Job drawing, mm, ordinate dimensions from the low corner. One solid piece. Coordinates: 2 decimals unless noted, no trailing zeros. Loops run counter-clockwise (first coordinate to the right, second up) from the corner with the lowest first, then second, coordinate; pieces in that order, holes last. Notation, with made-up numbers: (-29.5, 75.5) -> (11.5, 75.5) arc R6 ccw to (11.5, 86.5) -> close; hole circle Ø1 at (57, -36). An arc over 180 degrees is marked (long way). Use one line per item in the form item = value. Start each with the question number.
(1) Drill centre lines: L1, parallel to X at y = 21, z = 2.4; L2, parallel to Z at x = 17, y = 88. Where is each one in solid material? Low to high. Write a range as [from, to].
(2) Pin check, flat tips, straight feed: P1, Ø12, axis at x = 16, y = 41.5, coming from the +Z side; P2, Ø1, axis at x = 39.5, z = 3, coming from the +Y side; P3, Ø0.6, axis at x = 39.5, z = 2.5, coming from the -Y side. Stop position of each tip, or through.
(3) Band-saw the part on A-A on z = 2.85. Give the cut face in (x, y), then the cut area to 3 significant figures.
(4) Band-saw the part on B-B on y = 89.5. Give the cut face in (x, z).
(5) Band-saw the part on C-C on x = 25. Give the cut face in (y, z), then the cut area to 3 significant figures.
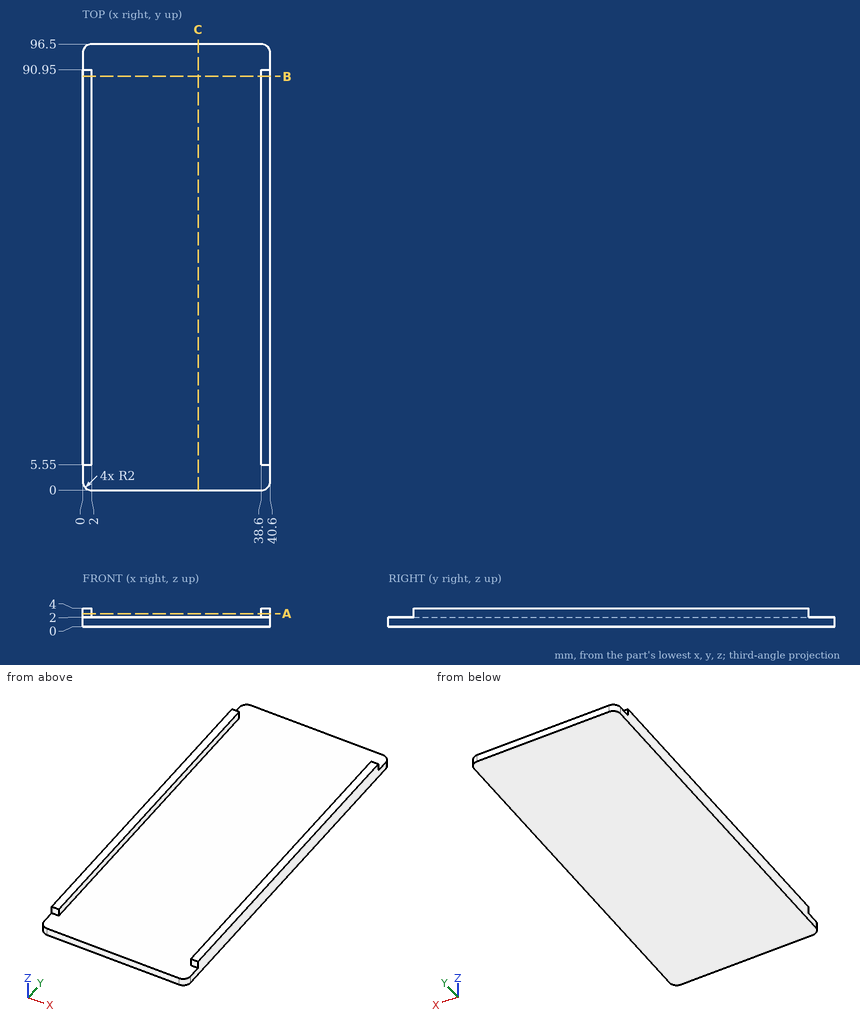
A:
q1.L1 = [0, 2], [38.6, 40.6]
q1.L2 = [0, 2]
q2.P1 = 2
q2.P2 = 90.95
q2.P3 = 5.55
q3.outline = (0, 5.55) -> (2, 5.55) -> (2, 90.95) -> (0, 90.95) -> close; (38.6, 5.55) -> (40.6, 5.55) -> (40.6, 90.95) -> (38.6, 90.95) -> close
q3.area = 342 mm²
q4.outline = (0, 0) -> (40.6, 0) -> (40.6, 4) -> (38.6, 4) -> (38.6, 2) -> (2, 2) -> (2, 4) -> (0, 4) -> close
q5.outline = (0, 0) -> (96.5, 0) -> (96.5, 2) -> (0, 2) -> close
q5.area = 193 mm²
